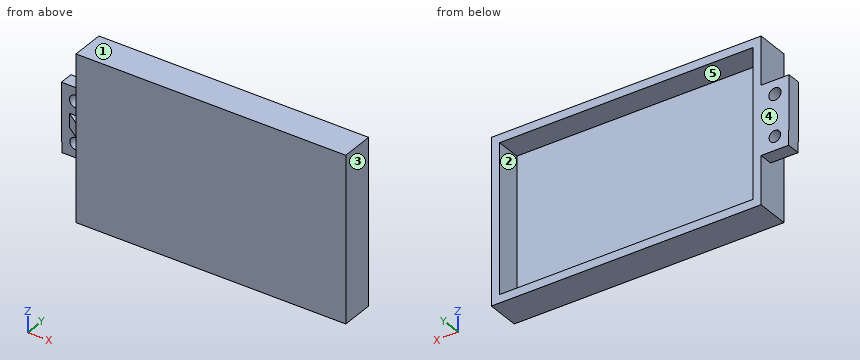
```python
from build123d import *

# Parameters (mm, degrees)
SKETCH_1_R          = 2.1
SKETCH_1_R_2        = 2.220092539
EXTRUDE_1_DEPTH     = 12
SKETCH_2_W          = 92
SKETCH_2_H          = 54
CUT_EXTRUDE_1_DEPTH = 9
SKETCH_3_W          = 10.168078989
SKETCH_3_H          = 25
CUT_EXTRUDE_2_DEPTH = 7
RIB_1_REACH         = 69.416
SKETCH_5_WALL_W     = 145.707888858
SKETCH_5_WALL_H     = 5


with BuildPart() as part:
    # 草图1 → 凸台-拉伸1 (new body)
    with BuildSketch(Plane(origin=(0, 0, 0), x_dir=(1, 0, 0), z_dir=(0, 1, 0))):
        Polygon((49, -30), (-49, -30), (-49, -12.5), (-59.168078989, -12.5), (-59, 12.5), (-49, 12.5), (-49, 30), (49, 30), align=None)
        with Locations(Location((-54, 7.5, 0), (0, 0, 270))):
            Circle(SKETCH_1_R, mode=Mode.SUBTRACT)
        with Locations(Location((-54, -7.5, 0), (0, 0, 270))):
            Circle(SKETCH_1_R_2, mode=Mode.SUBTRACT)
    extrude(amount=EXTRUDE_1_DEPTH)

    # 草图2 → 切除-拉伸1 (cut)
    with BuildSketch(Plane(origin=(0, 12, 0), x_dir=(1, 0, 0), z_dir=(0, 1, 0))):
        Rectangle(SKETCH_2_W, SKETCH_2_H)
    extrude(amount=-CUT_EXTRUDE_1_DEPTH, mode=Mode.SUBTRACT)

    # 草图3 → 切除-拉伸2 (cut)
    with BuildSketch(Plane.XZ):
        with Locations((-54.084039495, 0)):
            Rectangle(SKETCH_3_W, SKETCH_3_H)
    extrude(amount=-CUT_EXTRUDE_2_DEPTH, mode=Mode.SUBTRACT)

    # 草图5 wall → 筋1 (add, up to next)
    with BuildSketch(Plane(origin=(-52.61004627, 4.418029941, 0), x_dir=(0.813374663447, -0.581740197049, 0), z_dir=(0.581740197049, 0.813374663447, 0)), mode=Mode.PRIVATE) as rib_1_sk1:
        Rectangle(SKETCH_5_WALL_W, SKETCH_5_WALL_H)
    rib_1_tool1 = extrude(rib_1_sk1.sketch, amount=RIB_1_REACH, mode=Mode.PRIVATE) - part.part
    add(rib_1_tool1.solids().sort_by_distance((-52.61004627, 4.418029941, 0))[0])


solid = part.part
```
Work out the finished part from the listing and answer in its coordinate system (mm). Face numbers are marked on the shaded views. A direction names the side the tool comes from. Round coordinates to 2 decimals unless told otherwise and drop trailing zeros. Loops run counter-clockwise (first coordinate to the right, second up) from the corner with the lowest first, then second, coordinate; pieces in that order, holes last. Notation, with made-up numbers: (20, 55) -> (60, 55) arc R24 cw to (60, 79) -> close; hole circle Ø7 at (21.25, 26). An arc over 180 degrees is marked (long way). Write each question's results on one line, items separated by ' | '. Start each with the question number.
1. Given pin 1 Ø3 at (y, z) = (8, -6) entering from -X; pin 2 Ø2.5 at (y, z) = (9.5, -12.5) entering from -X; pin 3 Ø1 at (x, z) = (28.5, -17.5) entering from +Y, each flat-ended and moving along its own axis, determine where each tip first touches the part or whether it passes through.
2. For a pull along X with two mould halves and no side action, classify the marked faces 1, 2 and 3 as +X half, -X half, draft (parallel to the pull), parting line (faces both ways), or undercut.
3. Section D-D (y = 4.25) is taken. Determine the outline of the cut face in (x, z), plus the area to 3 significant figures.
4. Find the intervals of material crossed by probe 1 along Z at (x, y) = (-54, 9.35); probe 2 along Z at (x, y) = (-7.5, 5.25); probe 3 along X at (y, z) = (11.25, -26), in increasing order. Write a range as from..to.
5. A tool of negligible diameter and unlimited length cuts with its end or side. For the marked faces 4 and 5, from which of +Z, -Z, +X, -X, +Y, -Y can it reach the whole face along a straight path? Write none if from no direction.
6. Section A-A (y = 10.5) is taken. Determine the outline of the cut face in (x, z), plus the area to 3 significant figures.
7. Section B-B (z = 19) is taken. Determine the outline of the cut face in (x, y).
8. Section C-C (x = 29.5) is taken. Determine the outline of the cut face in (y, z).
Evaluation:
1) pin 1: stops at x = -59.05 | pin 2: stops at x = -59.01 | pin 3: stops at y = 3
2) face 1: draft | face 2: undercut | face 3: +X half
3) outline: (-52.38, -2.5) -> (-49, -2.5) -> (-49, -30) -> (49, -30) -> (49, 30) -> (-49, 30) -> (-49, 2.5) -> (-52.38, 2.5) -> close; hole (-46, -27) -> (46, -27) -> (46, 27) -> (-46, 27) -> close | area: 929 mm2
4) probe 1: z = -12.5..-9.6, -5.4..5.28, 9.72..12.5 | probe 2: z = -30..-27, 27..30 | probe 3: x = -49..-46, 46..49
5) face 4: +Z, -Z, +X, -X, +Y | face 5: +Y
6) outline: (-59.17, 12.5) -> (-59, -12.5) -> (-49, -12.5) -> (-49, -30) -> (49, -30) -> (49, 30) -> (-49, 30) -> (-49, 12.5) -> close; hole circle Ø4.44 at (-54, 7.5); hole circle Ø4.2 at (-54, -7.5); hole (-46, -27) -> (46, -27) -> (46, 27) -> (-46, 27) -> close | area: 1,130 mm2
7) outline: (-49, 0) -> (49, 0) -> (49, 12) -> (46, 12) -> (46, 3) -> (-46, 3) -> (-46, 12) -> (-49, 12) -> close
8) outline: (0, -30) -> (12, -30) -> (12, -27) -> (3, -27) -> (3, 27) -> (12, 27) -> (12, 30) -> (0, 30) -> close
